```python
from build123d import *

# Parameters (mm, degrees)
F0_W     = 152.4
F0_H     = 50.8
F1_DEPTH = 25.4
F2_R     = 15.875
F3_DEPTH = 25.4
F5_DEPTH = 6.35
F6_R     = 6.35


with BuildPart() as f1:
    # F0 (on Top) → F1 (new body)
    with BuildSketch(Plane.XY):
        Polygon((0, 127), (0, 0), (406.4, 0), (406.4, 304.8), (0, 304.8), (0, 177.8), align=None)
        with Locations((-76.2, 152.4)):
            Rectangle(F0_W, F0_H)
    extrude(amount=F1_DEPTH)

    # F2 (on face) → F3 (cut)
    with BuildSketch(Plane.XY.offset(25.4)):
        with Locations((-122.649528, 155.575)):
            Circle(F2_R)
    extrude(amount=-F3_DEPTH, mode=Mode.SUBTRACT)

    # F4 (on face) → F5 (cut)
    with BuildSketch(Plane.XY.offset(25.4)):
        Polygon((19.304004, 127), (19.304004, 19.304004), (387.095996, 19.304004), (387.095996, 285.495996), (19.304004, 285.495996), (19.304004, 177.8), align=None)
        Polygon((34.036007, 127), (34.036007, 177.8), (34.036007, 270.763993), (372.363993, 270.763993), (372.363993, 34.036007), (34.036007, 34.036007), align=None, mode=Mode.SUBTRACT)
    extrude(amount=-F5_DEPTH, mode=Mode.SUBTRACT)

    # F6
    f6_edges = [f1.edges().sort_by_distance(p)[0] for p in [
        (19.304004, 285.495996, 22.225),
        (387.095996, 285.495996, 22.225),
    ]]
    fillet(f6_edges, radius=F6_R)


solid = f1.part
```
Geometry: final body of the model. Coordinates: model frame, mm. A direction names the side the tool comes from. Round coordinates to 2 decimals unless told otherwise and drop trailing zeros. Write each loop counter-clockwise with the first axis right and the second up, starting at its lowest first coordinate (ties: lowest second). Pieces come first, ordered by that corner, then holes.
Item 1: Mould query, pull axis X, two halves, no side actions, for faces 1 (the face through (406.4, 150, 13)), 2 (the face through (0, 64, 13)), 3 (the face through (-115.324, 141.491, 12.878)), 4 (the face through (146, 18, 25.4)). Classes: +X half, -X half, draft (parallel to the pull), parting line (faces both ways), or undercut.
Item 2: Material intervals for L1, parallel to X at y = 46, z = 23.5; L2, parallel to Y at x = 375.5, z = 22.5; L3, parallel to Z at x = 28, y = 178.5, sorted ascending.
Item 3: Pin query (flat end, axial travel): P1, Ø12.5, axis at y = 46.5, z = 9, coming from the -X side. Return the tip coordinate at first contact, or that it passes through.
Item 4: Set-up query: faces 5 (the face through (0, 242, 13)), 6 (the face through (-77, 127, 13)), 7 (the face through (200, 0, 13)). Return all of +Z, -Z, +X, -X, +Y, -Y with unobstructed straight access to the full face (end or side cutting, diameter ignored); none if empty.
Item 5: Section query A-A (z = 9.25). Return loops of the section in (x, y) (3 decimals), plus the area to 3 significant figures.
Item 6: Section query D-D (x = -78.5). Return loops of the section in (y, z), plus the area to 3 significant figures.
Item 7: Section query C-C (x = 333). Return loops of the section in (y, z).
Item 8: Section query B-B (y = 218.5). Return loops of the section in (x, z).
Completed:
1. face 1: +X half
1. face 2: -X half
1. face 3: undercut
1. face 4: draft
2. L1: x = 0 to 19.3, 34.04 to 372.36, 387.1 to 406.4
2. L2: y = 0 to 19.3, 285.5 to 304.8
2. L3: z = 0 to 19.05
3. P1: stops at x = 0
4. face 5: +Z, -Z, -X, +Y
4. face 6: +Z, -Z, -X, -Y
4. face 7: +Z, -Z, +X, -X, -Y
5. outline: (-152.4, 127) - (0, 127) - (0, 0) - (406.4, 0) - (406.4, 304.8) - (0, 304.8) - (0, 177.8) - (-152.4, 177.8) - close; hole circle Ø31.75 at (-122.65, 155.575)
5. area: 131,000 mm2
6. outline: (127, 0) - (177.8, 0) - (177.8, 25.4) - (127, 25.4) - close
6. area: 1,290 mm2
7. outline: (0, 0) - (304.8, 0) - (304.8, 25.4) - (285.5, 25.4) - (285.5, 19.05) - (270.76, 19.05) - (270.76, 25.4) - (34.04, 25.4) - (34.04, 19.05) - (19.3, 19.05) - (19.3, 25.4) - (0, 25.4) - close
8. outline: (0, 0) - (406.4, 0) - (406.4, 25.4) - (387.1, 25.4) - (387.1, 19.05) - (372.36, 19.05) - (372.36, 25.4) - (34.04, 25.4) - (34.04, 19.05) - (19.3, 19.05) - (19.3, 25.4) - (0, 25.4) - close
